```python
from build123d import *

# Parameters (mm, degrees)
BOSS_EXTRUDE1_DEPTH = 5
SKETCH2_R           = 2.5
CUT_EXTRUDE1_DEPTH  = 5


with BuildPart() as part:
    # Sketch1 → Boss-Extrude1 (new body)
    with BuildSketch(Plane(origin=(0, 0, 0), x_dir=(1, 0, 0), z_dir=(0, 1, 0))):
        with BuildLine():
            ThreePointArc((11.892024371, 4.925837778), (12.551145366, 12.551145366), (4.925837778, 11.892024371))
            ThreePointArc((4.925837778, 11.892024371), (0, 7.75), (-4.925837778, 11.892024371))
            ThreePointArc((-4.925837778, 11.892024371), (-12.551145366, 12.551145366), (-11.892024371, 4.925837778))
            ThreePointArc((-11.892024371, 4.925837778), (-7.75, 0), (-11.892024371, -4.925837778))
            ThreePointArc((-11.892024371, -4.925837778), (-12.551145366, -12.551145366), (-4.925837778, -11.892024371))
            ThreePointArc((-4.925837778, -11.892024371), (0, -7.75), (4.925837778, -11.892024371))
            ThreePointArc((4.925837778, -11.892024371), (12.551145366, -12.551145366), (11.892024371, -4.925837778))
            ThreePointArc((11.892024371, -4.925837778), (7.75, 0), (11.892024371, 4.925837778))
        make_face()
    extrude(amount=BOSS_EXTRUDE1_DEPTH)

    # Sketch2 → Cut-Extrude1 (cut)
    with BuildSketch(Plane(origin=(0, 5, 0), x_dir=(1, 0, 0), z_dir=(0, 1, 0))):
        Circle(SKETCH2_R)
    extrude(amount=-CUT_EXTRUDE1_DEPTH, mode=Mode.SUBTRACT)


solid = part.part
```
Could you check a few things on this model? Use its own coordinates, in mm. Round coordinates to 2 decimals unless told otherwise and drop trailing zeros. Loops run counter-clockwise (first coordinate to the right, second up) from the corner with the lowest first, then second, coordinate; pieces in that order, holes last.
Q1. I want a section at A-A (x = 0). Write out the boundary of the cut face in (y, z).
Q2. Thinking about a two-plate mould opening in Z: for faces 1 (the cylindrical face through (-12.6, 2.5, 12.5)), 2 (the flat face through (0, 0, 3)), 3 (the cylindrical face through (-0.1, 2.46, 7.75)), which applies, pulls with the +Z half, pulls with the -Z half, needs draft (parallel to the pull), parting line crosses it, or undercut?
Q3. I want a section at D-D (z = 4.25). Write out the boundary of the cut face in (x, y), and give its area (3 significant figures).
Q4. For P1, Ø1, axis at x = 0.5, y = 3.5, coming from the -Z side; P2, Ø10, axis at x = 10.5, z = -6.5, coming from the -Y side; P3, Ø1, axis at x = -4, y = 4, coming from the -Z side; P4, Ø2, axis at y = 2, z = 1, coming from the +X side, each with a flat end and sliding along its axis, tell me the tip position at first contact or that it passes through.
Q5. Please list where these lines run through material, in increasing order: L1, parallel to X at y = 1.05, z = 10.5; L2, parallel to Z at x = -9.5, y = 3.55; L3, parallel to Z at x = -0.75, y = 4.65.
Q6. I want a section at C-C (y = 0.5). Write out the boundary of the cut face in (x, z), and give its area (3 significant figures).
Q7. I want a section at B-B (z = 0). Write out the boundary of the cut face in (x, y).
Answer below:
1. outline: (0, -7.75) - (5, -7.75) - (5, -2.5) - (0, -2.5) - close; (0, 2.5) - (5, 2.5) - (5, 7.75) - (0, 7.75) - close
2. face 1: undercut
2. face 2: needs draft
2. face 3: pulls with the +Z half
3. outline: (-10.12, 0) - (10.12, 0) - (10.12, 5) - (-10.12, 5) - close
3. area: 101 mm2
4. P1: stops at z = -7.85
4. P2: stops at y = 0
4. P3: stops at z = -10.57
4. P4: stops at x = 8.17
5. L1: x = -13.79 to -4.47, 4.47 to 13.79
5. L2: z = -13.99 to -3.8, 3.8 to 13.99
5. L3: z = -7.81 to -2.38, 2.38 to 7.81
6. outline: (-11.89, -4.93) arc R5 ccw (long way) to (-4.93, -11.89) arc R5 cw to (4.93, -11.89) arc R5 ccw (long way) to (11.89, -4.93) arc R5 cw to (11.89, 4.93) arc R5 ccw (long way) to (4.93, 11.89) arc R5 cw to (-4.93, 11.89) arc R5 ccw (long way) to (-11.89, 4.93) arc R5 cw to start; hole circle Ø5 at (0, 0)
6. area: 517 mm2
7. outline: (-7.75, 0) - (-2.5, 0) - (-2.5, 5) - (-7.75, 5) - close; (2.5, 0) - (7.75, 0) - (7.75, 5) - (2.5, 5) - close
